Check sheet for the modelled part. Datum: model origin and axes. Units: mm. A direction names the side the tool comes from. Round coordinates to 2 decimals unless told otherwise and drop trailing zeros. Order: outer loops, then holes, each group sorted by start corner. A loop starts at its lowest first (then second) coordinate and runs counter-clockwise, first axis right, second up. Notation, with made-up numbers: (22.25, 4) -> (75.25, 4) arc R7 cw to (75.25, 9) -> close; hole circle Ø11 at (37, -28.75). An arc over 180 degrees is marked (long way). Answer in a Markdown table with one row per item.
```python
from build123d import *

# Parameters (mm, degrees)
CYLINDER282_R               = 3
CYLINDER282_DEPTH           = 12
BOX184_W                    = 16
BOX184_H                    = 7.5
BOX184_DEPTH                = 12
CYLINDER271_R               = 2
CYLINDER271_DEPTH           = 15
BOX185_W                    = 22
BOX185_H                    = 12
BOX185_DEPTH                = 10
FILLET120_R                 = 4.9
FILLET120_PLACEMENT_ANGLE   = 180
CHAMFER035_SIZE             = 6.5
CYLINDER275_R               = 1.5
CYLINDER275_DEPTH           = 18
BOX194_W                    = 2
BOX194_H                    = 8.89
BOX194_DEPTH                = 21.59
FUSION188_PLACEMENT_ANGLE   = 20
CYLINDER276_R               = 1.5
CYLINDER276_DEPTH           = 18
BOX195_W                    = 2
BOX195_H                    = 8.89
BOX195_DEPTH                = 21.59
FUSION189_PLACEMENT_ANGLE   = 20
CYLINDER272_R               = 1.5
CYLINDER272_DEPTH           = 18
BOX186_W                    = 2
BOX186_H                    = 8.89
BOX186_DEPTH                = 21.59
CYLINDER280_R               = 3
CYLINDER280_DEPTH           = 12
CYLINDER281_R               = 3
CYLINDER281_DEPTH           = 8
CYLINDER281_PITCH_ANGLE     = 90
CYLINDER281_PLACEMENT_ANGLE = 20
CYLINDER279_R               = 3
CYLINDER279_DEPTH           = 8
CYLINDER279_PITCH_ANGLE     = 90
CYLINDER279_PLACEMENT_ANGLE = 20
BOX190_W                    = 10
BOX190_H                    = 10
BOX190_DEPTH                = 12
BOX191_W                    = 10
BOX191_H                    = 10
BOX191_DEPTH                = 12
BOX189_W                    = 62
BOX189_H                    = 73
BOX189_DEPTH                = 12
TUBE_R                      = 35
TUBE_R_2                    = 28
TUBE_DEPTH                  = 10
FUSION196_PLACEMENT_ANGLE   = 20


with BuildPart() as zylinder284:
    # Cylinder282 → Cylinder282 (new body)
    with BuildSketch(Plane(origin=(44, 0, -11.55), x_dir=(0, 0, -1), z_dir=(1, 0, 0))):
        Circle(CYLINDER282_R)
    extrude(amount=CYLINDER282_DEPTH)


with BuildPart() as obj1:
    # Box184 → Box184 (new body)
    with BuildSketch(Plane(origin=(28.5, -3.75, -11.5), x_dir=(1, 0, 0), z_dir=(0, 0, 1))):
        with Locations((8, 3.75)):
            Rectangle(BOX184_W, BOX184_H)
    extrude(amount=BOX184_DEPTH)


with BuildPart() as fusion185:
    # Cylinder271 → Cylinder271 (new body)
    with BuildSketch(Plane(origin=(37.5, 7.5, -5.5), x_dir=(1, 0, 0), z_dir=(0, -1, 0))):
        Circle(CYLINDER271_R)
    extrude(amount=CYLINDER271_DEPTH)

    # Fusion185: union obj1
    add(obj1.part)


with BuildPart() as cut132:
    # Box185 → Box185 (new body)
    with BuildSketch(Plane(origin=(27, -3.5, -10.5), x_dir=(1, 0, 0), z_dir=(0, 0, 1))):
        with Locations((11, 6)):
            Rectangle(BOX185_W, BOX185_H)
    extrude(amount=BOX185_DEPTH)

    # Fillet120
    fillet120_edges = [cut132.edges().sort_by_distance(p)[0] for p in [
        (49, 2.5, -0.5),
        (49, 2.5, -10.5),
    ]]
    fillet(fillet120_edges, radius=FILLET120_R)


with BuildPart() as cut132_1:
    # Fillet120 placement: moved
    add(cut132.part.moved(Location((82, -2.5, -11))).rotate(Axis((82, -2.5, -11), (0, 1, 0)), FILLET120_PLACEMENT_ANGLE))

    # Cut122: cut Fusion185
    add(fusion185.part, mode=Mode.SUBTRACT)

    # Chamfer035
    chamfer035_edges = [cut132_1.edges().sort_by_distance(p)[0] for p in [
        (55, 0, -0.5),
    ]]
    chamfer(chamfer035_edges, length=CHAMFER035_SIZE)

    # Cut132: cut Zylinder284
    add(zylinder284.part, mode=Mode.SUBTRACT)


with BuildPart() as zylinder277:
    # Cylinder275 → Cylinder275 (new body)
    with BuildSketch(Plane(origin=(48, 0, -11.55), x_dir=(0, 0, -1), z_dir=(1, 0, 0))):
        Circle(CYLINDER275_R)
    extrude(amount=CYLINDER275_DEPTH)


with BuildPart() as fusion188:
    # Box194 → Box194 (new body)
    with BuildSketch(Plane(origin=(61.5, -4.5, -14), x_dir=(1, 0, 0), z_dir=(0, 0, 1))):
        with Locations((1, 4.445)):
            Rectangle(BOX194_W, BOX194_H)
    extrude(amount=BOX194_DEPTH)

    # Fusion188: union Zylinder277
    add(zylinder277.part)


with BuildPart() as fusion188_1:
    # Fusion188 placement: moved
    add(fusion188.part.moved(Location((-0.210743, 9.654304, 0))).rotate(Axis((-0.210743, 9.654304, 0), (0, 0, -1)), FUSION188_PLACEMENT_ANGLE))


with BuildPart() as zylinder278:
    # Cylinder276 → Cylinder276 (new body)
    with BuildSketch(Plane(origin=(48, 0, -11.55), x_dir=(0, 0, -1), z_dir=(1, 0, 0))):
        Circle(CYLINDER276_R)
    extrude(amount=CYLINDER276_DEPTH)


with BuildPart() as fusion189:
    # Box195 → Box195 (new body)
    with BuildSketch(Plane(origin=(61.5, -4.5, -14), x_dir=(1, 0, 0), z_dir=(0, 0, 1))):
        with Locations((1, 4.445)):
            Rectangle(BOX195_W, BOX195_H)
    extrude(amount=BOX195_DEPTH)

    # Fusion189: union Zylinder278
    add(zylinder278.part)


with BuildPart() as fusion189_1:
    # Fusion189 placement: moved
    add(fusion189.part.moved(Location((-0.210743, 9.654304, 0))).rotate(Axis((-0.210743, 9.654304, 0), (0, 0, -1)), FUSION189_PLACEMENT_ANGLE))


with BuildPart() as part_mirroring007:
    # Part__Mirroring007: instance of Fusion189
    add(fusion189_1.part.mirror(Plane(origin=(0, 0, 0), x_dir=(1, 0, 0), z_dir=(0, 1, 0))))


with BuildPart() as zylinder274:
    # Cylinder272 → Cylinder272 (new body)
    with BuildSketch(Plane(origin=(48, 0, -11.55), x_dir=(0, 0, -1), z_dir=(1, 0, 0))):
        Circle(CYLINDER272_R)
    extrude(amount=CYLINDER272_DEPTH)


with BuildPart() as fusion193:
    # Box186 → Box186 (new body)
    with BuildSketch(Plane(origin=(61.5, -4.5, -14), x_dir=(1, 0, 0), z_dir=(0, 0, 1))):
        with Locations((1, 4.445)):
            Rectangle(BOX186_W, BOX186_H)
    extrude(amount=BOX186_DEPTH)

    # Fusion187: union Zylinder274
    add(zylinder274.part)


with BuildPart() as fusion193_1:
    # Fusion187 placement: moved
    add(fusion193.part.moved(Location((-2, 0, 0))))

    # Fusion193: union Fusion188, Part__Mirroring007
    add(fusion188_1.part)
    add(part_mirroring007.part)


with BuildPart() as zylinder282:
    # Cylinder280 → Cylinder280 (new body)
    with BuildSketch(Plane(origin=(44, 0, -11.55), x_dir=(0, 0, -1), z_dir=(1, 0, 0))):
        Circle(CYLINDER280_R)
    extrude(amount=CYLINDER280_DEPTH)


with BuildPart() as zylinder283:
    # Cylinder281 → Cylinder281 (new body)
    with BuildSketch(Plane.XY):
        Circle(CYLINDER281_R)
    extrude(amount=CYLINDER281_DEPTH)


with BuildPart() as zylinder283_1:
    # Cylinder281 pitch: moved
    add(zylinder283.part.rotate(Axis((0, 0, 0), (0, 1, 0)), CYLINDER281_PITCH_ANGLE))


with BuildPart() as zylinder283_2:
    # Cylinder281 placement: moved
    add(zylinder283_1.part.moved(Location((46.763839, 7.517541, -11.55))).rotate(Axis((46.763839, 7.517541, -11.55), (0, 0, 1)), CYLINDER281_PLACEMENT_ANGLE))


with BuildPart() as zylinder281:
    # Cylinder279 → Cylinder279 (new body)
    with BuildSketch(Plane.XY):
        Circle(CYLINDER279_R)
    extrude(amount=CYLINDER279_DEPTH)


with BuildPart() as zylinder281_1:
    # Cylinder279 pitch: moved
    add(zylinder281.part.rotate(Axis((0, 0, 0), (0, 1, 0)), CYLINDER279_PITCH_ANGLE))


with BuildPart() as zylinder281_2:
    # Cylinder279 placement: moved
    add(zylinder281_1.part.moved(Location((46.763839, 7.517541, -11.55))).rotate(Axis((46.763839, 7.517541, -11.55), (0, 0, 1)), CYLINDER279_PLACEMENT_ANGLE))


with BuildPart() as fusion195:
    # Part__Mirroring009: instance of Zylinder281
    add(zylinder281_2.part.mirror(Plane(origin=(0, 0, 0), x_dir=(1, 0, 0), z_dir=(0, 1, 0))))

    # Fusion195: union Zylinder282, Zylinder283
    add(zylinder282.part)
    add(zylinder283_2.part)


with BuildPart() as obj2:
    # Box190 → Box190 (new body)
    with BuildSketch(Plane(origin=(47.5, -27.5, -18), x_dir=(1, 0, 0), z_dir=(0, 0, 1))):
        with Locations((5, 5)):
            Rectangle(BOX190_W, BOX190_H)
    extrude(amount=BOX190_DEPTH)


with BuildPart() as obj3:
    # Box191 → Box191 (new body)
    with BuildSketch(Plane(origin=(47.5, 17.5, -18), x_dir=(1, 0, 0), z_dir=(0, 0, 1))):
        with Locations((5, 5)):
            Rectangle(BOX191_W, BOX191_H)
    extrude(amount=BOX191_DEPTH)


with BuildPart() as fusion186:
    # Box189 → Box189 (new body)
    with BuildSketch(Plane(origin=(-10.5, -37, -18), x_dir=(1, 0, 0), z_dir=(0, 0, 1))):
        with Locations((31, 36.5)):
            Rectangle(BOX189_W, BOX189_H)
    extrude(amount=BOX189_DEPTH)

    # Fusion186: union obj2, obj3
    add(obj2.part)
    add(obj3.part)


with BuildPart() as obj4:
    # Tube → Tube (new body)
    with BuildSketch(Plane(origin=(25.5, 0, -17), x_dir=(1, 0, 0), z_dir=(0, 0, 1))):
        Circle(TUBE_R)
        Circle(TUBE_R_2, mode=Mode.SUBTRACT)
    extrude(amount=TUBE_DEPTH)

    # Cut126: cut Fusion186
    add(fusion186.part, mode=Mode.SUBTRACT)

    # Cut130: cut Fusion195
    add(fusion195.part, mode=Mode.SUBTRACT)

    # Cut131: cut Fusion193
    add(fusion193_1.part, mode=Mode.SUBTRACT)

    # Fusion196: union Cut132
    add(cut132_1.part)


with BuildPart() as obj4_1:
    # Fusion196 placement: moved
    add(obj4.part.moved(Location((4.168672, 0, 12.476665))).rotate(Axis((4.168672, 0, 12.476665), (0, 1, 0)), FUSION196_PLACEMENT_ANGLE))


solid = obj4_1.part
```
(1) Tool access check on faces 4 (the flat face through (51.2, -9.04, -18.31)), 5 (the flat face through (56.362, -7.364, -17.746)), 6 (the flat face through (53.53, 15.73, -16.72)), 7 (the flat face through (48.435, 13.896, -16.479)). Record the directions out of +Z, -Z, +X, -X, +Y, -Y that give a thin tool (end or side, any length) a straight path to the whole face; none if there is none.
Solutions:
| item | result |
|---|---|
| face 4 | none |
| face 5 | -Y |
| face 6 | +X |
| face 7 | +Z, -X, +Y |
(2) Scan lines: probe 1 along Y at (x, z) = (42.75, -5); probe 2 along X at (y, z) = (12, -18.75); probe 3 along Y at (x, z) = (56.5, -17.5). Record each from-to range of solid material in increasing order. Write a range as from..to.
Solutions:
| item | result |
|---|---|
| probe 1 | -6..-3.75, 3.75..6 |
| probe 2 | 47.61..49.56, 49.89..52.86 |
| probe 3 | -7.38..-0.78, 0.78..7.38 |
(3) Depth check by flat-ended pin: pin 1 Ø6 at (y, z) = (1.5, -19) entering from +X; pin 2 Ø10 at (y, z) = (-6, -4) entering from -X; pin 3 Ø12 at (x, z) = (38, -8.5) entering from +Y; pin 4 Ø8 at (y, z) = (-10.5, -17.5) entering from +X. Enter the tip coordinate at first touch or a pass-through.
Solutions:
| item | result |
|---|---|
| pin 1 | x = 57.12 |
| pin 2 | x = 32.97 |
| pin 3 | y = 6 |
| pin 4 | x = 57.73 |
(4) Section check D-D on z = -8.5. Record the boundary of the cut face in (x, y).
Solutions:
| item | result |
|---|---|
| outline | (33.81, -6) -> (51.4, -6) -> (51.4, 6) -> (33.81, 6) -> (33.81, 3.75) -> (43.89, 3.75) -> (43.89, -3.75) -> (33.81, -3.75) -> close |
(5) Section check C-C on y = 14. Record the boundary of the cut face in (x, z).
Solutions:
| item | result |
|---|---|
| outline | (46.75, -21.11) -> (52.46, -23.19) -> (53.49, -20.37) -> (52.59, -20.05) -> (54.99, -13.47) -> (50.17, -11.72) -> close |
(6) Draft check along X on faces 1 (the flat face through (54.21, 0.245, -13.186)), 2 (the cylindrical face through (39.524, -4.859, -5.605)), 3 (the flat face through (50.92, 0.24, -22.63)). Enter one of: pulls with the +X half, pulls with the -X half, needs draft (parallel to the pull), parting line crosses it, or undercut.
Solutions:
| item | result |
|---|---|
| face 1 | pulls with the +X half |
| face 2 | undercut |
| face 3 | pulls with the -X half |
(7) Section check A-A on z = -5.75. Record the boundary of the cut face in (x, y), plus the area to 3 significant figures.
Solutions:
| item | result |
|---|---|
| outline | (32.97, -6) -> (35.54, -6) -> (35.54, -3.75) -> (32.97, -3.75) -> close; (32.97, 3.75) -> (35.54, 3.75) -> (35.54, 6) -> (32.97, 6) -> close; (39.51, -6) -> (50.12, -6) -> (50.12, 6) -> (39.51, 6) -> (39.51, 3.75) -> (44.89, 3.75) -> (44.89, -3.75) -> (39.51, -3.75) -> close |
| area | 98.5 mm^2 |
(8) Section check B-B on y = -0.5. Record the boundary of the cut face in (x, z).
Solutions:
| item | result |
|---|---|
| outline | (43.05, -10.82) -> (53.85, -14.75) -> (53.32, -16.2) -> (56.61, -17.4) -> (57.69, -14.45) -> (53.46, -12.91) -> (49.57, -4.58) -> (45.81, -3.21) -> close; (48.62, -21.79) -> (55.2, -24.19) -> (56.23, -21.37) -> (55.29, -21.03) -> (55.65, -20.06) -> (52.36, -18.86) -> (51.83, -20.31) -> (49.48, -19.45) -> close |
